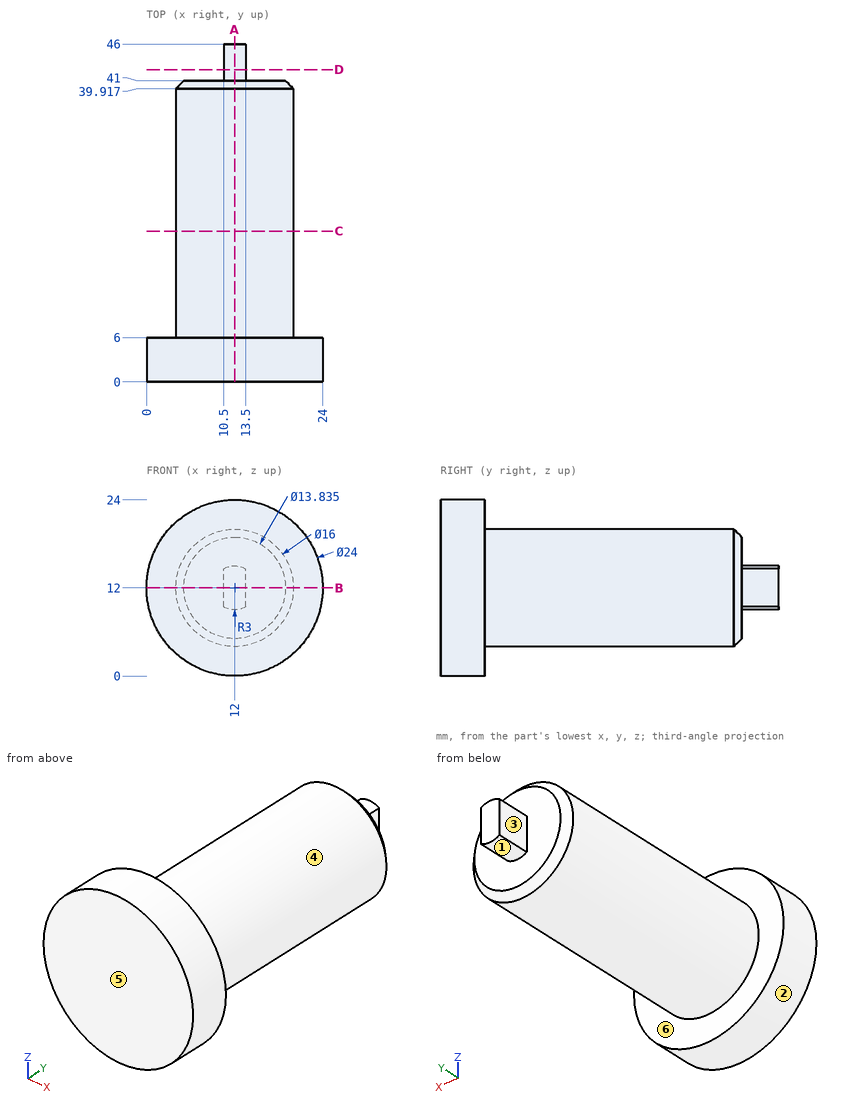
Verification items for this drawing (mm, ordinates from the low corner). A direction names the side the tool comes from. Coordinates: 2 decimals unless noted, no trailing zeros. Write each loop counter-clockwise with the first axis right and the second up, starting at its lowest first coordinate (ties: lowest second). Pieces come first, ordered by that corner, then holes. Notation, with made-up numbers: M 57.5,22.25 L 90.5,22.25 A21 cw 90.5,43.25 Z; hole C -0.75,41.5 d10. An arc over 180 degrees is marked long. Use one line per item in the form item = value. Start each with the question number.
1) Set-up check for the marked faces 1, 2 and 3: record each of +Z, -Z, +X, -X, +Y, -Y from which the full face is reachable in a straight line by a thin tool's end or side.
2) Release check for a two-part mould opening along Y. For the marked faces 4, 5 and 6 record: pulls with the +Y half, pulls with the -Y half, needs draft (parallel to the pull), parting line crosses it, or undercut.
3) Section check A-A on x = 12. Enter the section's corners in (y, z), and give its area (3 significant figures).
4) Section check B-B on z = 12. Enter the section's corners in (x, y), and give its area (3 significant figures).
5) Go/stop test with flat-tipped pins: pin 1 Ø6 at (x, y) = (5, 17.5) entering from -Z; pin 2 Ø5.5 at (y, z) = (44, 12.5) entering from -X; pin 3 Ø3 at (y, z) = (36.5, 9) entering from -X. Record where each tip stops, or that it passes through.
6) Section check C-C on y = 20.5. Enter the section's corners in (x, z), and give its area (3 significant figures).
7) Section check D-D on y = 42.5. Enter the section's corners in (x, z).
8) Thickness scan on probe 1 along Y at (x, z) = (9.75, 14.25); probe 2 along Y at (x, z) = (10, 22.25); probe 3 along X at (y, z) = (34.5, 12). Record the ranges inside material, lowest first. Write a range as from..to.
Responses:
q1.face_1 = -Z, +Y
q1.face_2 = +Y, -Y
q1.face_3 = +Z, -Z, -X, +Y
q2.face_4 = needs draft
q2.face_5 = pulls with the -Y half
q2.face_6 = pulls with the +Y half
q3.outline = M 0,0 L 6,0 L 6,4 L 39.92,4 L 41,5.08 L 41,9 L 46,9 L 46,15 L 41,15 L 41,18.92 L 39.92,20 L 6,20 L 6,24 L 0,24 Z
q3.area = 733 mm2
q4.outline = M 0,0 L 24,0 L 24,6 L 20,6 L 20,39.92 L 18.92,41 L 13.5,41 L 13.5,46 L 10.5,46 L 10.5,41 L 5.08,41 L 4,39.92 L 4,6 L 0,6 Z
q4.area = 718 mm2
q5.pin_1 = 5.07
q5.pin_2 = 10.5
q5.pin_3 = 4.14
q6.outline = C 12,12 d16
q6.area = 201 mm2
q7.outline = M 10.5,9.4 A3 ccw 13.5,9.4 L 13.5,14.6 A3 ccw 10.5,14.6 Z
q8.probe_1 = 0..41
q8.probe_2 = 0..6
q8.probe_3 = 4..20
